Input: part model. Units: mm. Frame: model coordinates. A direction names the side the tool comes from. Round coordinates to 2 decimals unless told otherwise and drop trailing zeros. Write each loop counter-clockwise with the first axis right and the second up, starting at its lowest first coordinate (ties: lowest second). Pieces come first, ordered by that corner, then holes. Notation, with made-up numbers: (-24, 77) - (3, 77) arc R29 ccw to (3, 99) - close; hole circle Ø3 at (67, 14). An arc over 180 degrees is marked (long way). Use one line per item in the form item = value.
```python
from build123d import *

# Parameters (mm, degrees)
SKETCH3_R           = 2.6035
CUT_EXTRUDE1_DEPTH  = 25.384
SKETCH4_R           = 24.384
SKETCH4_R_2         = 24.13
BOSS_EXTRUDE1_DEPTH = 2.54


with BuildPart() as part:
    # Sketch2 → Revolve1 (revolve)
    with BuildSketch(Plane(origin=(0, 0, 0), x_dir=(0, 0, -1), z_dir=(1, 0, 0))):
        with BuildLine():
            Line((24.13, 0), (24.384, 0))
            ThreePointArc((24.384, 0), (17.242091752, 17.242091752), (0, 24.384))
            Line((0, 24.384), (0, 24.13))
            ThreePointArc((0, 24.13), (17.06248663, 17.06248663), (24.13, 0))
        make_face()
    revolve(axis=Axis((0, 0, 0), (0, 1, 0)))

    # Sketch3 → Cut-Extrude1 (cut, through all)
    with BuildSketch(Plane(origin=(0, 0, 0), x_dir=(1, 0, 0), z_dir=(0, 1, 0))):
        Circle(SKETCH3_R)
    extrude(amount=CUT_EXTRUDE1_DEPTH, mode=Mode.SUBTRACT)

    # Sketch4 → Boss-Extrude1 (add)
    with BuildSketch(Plane(origin=(0, 0, 0), x_dir=(1, 0, 0), z_dir=(0, 1, 0))):
        Circle(SKETCH4_R)
        Circle(SKETCH4_R_2, mode=Mode.SUBTRACT)
    extrude(amount=-BOSS_EXTRUDE1_DEPTH)


solid = part.part
```
(1) Access query for faces 1 (the face through (23.016, -1.252, -7.248)), 2 (the face through (-3.174, -1.252, -24.177)). Directions: +Z, -Z, +X, -X, +Y, -Y. A direction counts if a zero-diameter tool reaches every point of the face in a straight line with its end or side. Return the directions, or none.
Derived:
face_1 = -Y
face_2 = +Y, -Y
(2) Material intervals for L1, parallel to X at y = -1, z = 0; L2, parallel to Z at x = -18, y = 0.75, sorted ascending.
Derived:
L1 = -24.38 to -24.13, 24.13 to 24.38
L2 = -16.43 to -16.05, 16.05 to 16.43
(3) Cut plane D-D on x = 20.5. Output: boundary loops of the cut face in (y, z), then the cut area to 3 significant figures.
Derived:
outline = (-2.54, -13.2) - (0, -13.2) arc R13.2 ccw to (0, 13.2) - (-2.54, 13.2) - (-2.54, 12.73) - (0, 12.73) arc R12.73 cw to (0, -12.73) - (-2.54, -12.73) - close
area = 21.8 mm^2
(4) Cut plane A-A on z = 0. Output: boundary loops of the cut face in (x, y), then the cut area to 3 significant figures.
Derived:
outline = (-24.38, -2.54) - (-24.13, -2.54) - (-24.13, 0) arc R24.13 cw to (-2.6, 23.99) - (-2.6, 24.24) arc R24.38 ccw to (-24.38, 0) - close; (2.6, 23.99) arc R24.13 cw to (24.13, 0) - (24.13, -2.54) - (24.38, -2.54) - (24.38, 0) arc R24.38 ccw to (2.6, 24.24) - close
area = 19.3 mm^2
(5) First-contact query: pin 1 Ø1 at (x, z) = (12.5, 13.5) entering from +Y; pin 2 Ø2 at (x, z) = (-12.5, -17.5) entering from +Y; pin 3 Ø3 at (x, z) = (0, 0) entering from +Y; pin 4 Ø1.5 at (y, z) = (3.5, 1.5) entering from -X. Flat tips, straight axial feed; report the tip coordinate or a pass-through.
Derived:
pin_1 = 16.56
pin_2 = 13.19
pin_3 = through
pin_4 = -24.19
(6) Cut plane B-B on x = 0. Output: boundary loops of the cut face in (y, z), then the cut area to 3 significant figures.
Derived:
outline = (-2.54, -24.38) - (0, -24.38) arc R24.38 ccw to (24.24, -2.6) - (23.99, -2.6) arc R24.13 cw to (0, -24.13) - (-2.54, -24.13) - close; (-2.54, 24.13) - (0, 24.13) arc R24.13 cw to (23.99, 2.6) - (24.24, 2.6) arc R24.38 ccw to (0, 24.38) - (-2.54, 24.38) - close
area = 19.3 mm^2
(7) Cut plane C-C on z = -13.5. Output: boundary loops of the cut face in (x, y), then the cut area to 3 significant figures.
Derived:
outline = (-20.31, -2.54) - (-20, -2.54) - (-20, 0) arc R20 cw to (20, 0) - (20, -2.54) - (20.31, -2.54) - (20.31, 0) arc R20.31 ccw to (-20.31, 0) - close
area = 20.9 mm^2
